Input: dimensioned drawing with shaded views. Units: mm. Origin: part minimum x, y, z. A direction names the side the tool comes from. Round coordinates to 2 decimals unless told otherwise and drop trailing zeros. Loops run counter-clockwise (first coordinate to the right, second up) from the corner with the lowest first, then second, coordinate; pieces in that order, holes last. Notation, with made-up numbers: M 43.5,-9 L 59.5,-9 A25 cw 59.5,6 Z; hole C 15,-35 d9. An arc over 180 degrees is marked long. Use one line per item in the form item = value. Start each with the question number.
Q1. Section query A-A, the plane x = 3.25. Output: boundary loops of the cut face in (y, z), and give its area (3 significant figures).
Q2. Section query C-C, the plane z = 1.85. Output: boundary loops of the cut face in (x, y).
Q3. First-contact query: P1, Ø0.7, axis at x = 3.5, z = 1, coming from the -Y side; P2, Ø0.7, axis at x = 3, z = 0.5, coming from the +Y side; P3, Ø1.5, axis at y = 3, z = 0.5, coming from the +X side; P4, Ø0.7, axis at y = 3.5, z = 1, coming from the -X side. Flat tips, straight axial feed; report the tip coordinate or a pass-through.
Q4. Section query D-D, the plane x = 5.75. Output: boundary loops of the cut face in (y, z), and give its area (3 significant figures).
Q5. Mould query, pull axis Y, two halves, no side actions, for the marked faces 6, 7, 8 and 9. Classes: pulls with the +Y half, pulls with the -Y half, needs draft (parallel to the pull), parting line crosses it, or undercut.
Q6. Access query for the marked faces 1, 2, 3, 4 and 5. Directions: +Z, -Z, +X, -X, +Y, -Y. A direction counts if a zero-diameter tool reaches every point of the face in a straight line with its end or side. Return the directions, or none.
Q7. Ray query, line 1 along Z through (x, y) = (2, 4.25); line 2 along Y through (x, z) = (3.75, 1.35); line 3 along X through (y, z) = (2.75, 1.5). Return the intervals inside material, ascending.
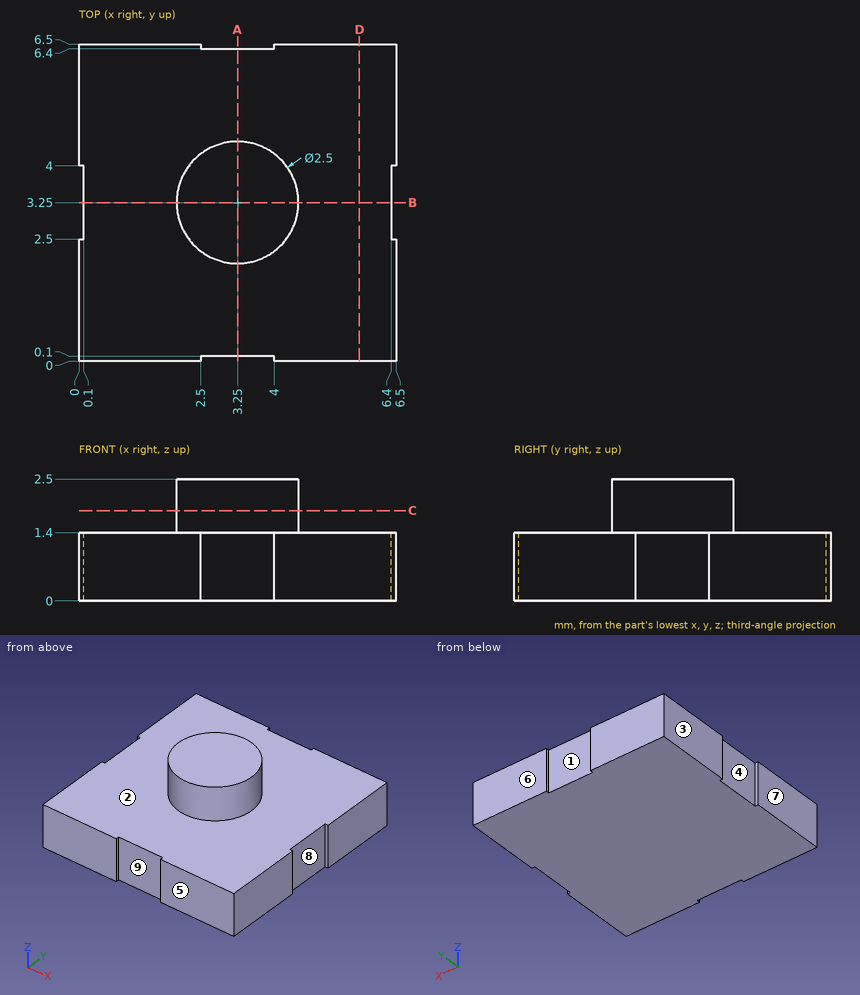
Results found:
q1.outline = M 0.1,0 L 6.4,0 L 6.4,1.4 L 4.5,1.4 L 4.5,2.5 L 2,2.5 L 2,1.4 L 0.1,1.4 Z
q1.area = 11.6 mm²
q2.outline = C 3.25,3.25 d2.5
q3.P1 = 0.1
q3.P2 = 6.4
q3.P3 = 6.5
q3.P4 = 0.1
q4.outline = M 0,0 L 6.5,0 L 6.5,1.4 L 0,1.4 Z
q4.area = 9.10 mm²
q5.face_6 = pulls with the +Y half
q5.face_7 = needs draft
q5.face_8 = undercut
q5.face_9 = pulls with the -Y half
q6.face_1 = +Z, -Z, +Y
q6.face_2 = +Z
q6.face_3 = +Z, -Z, -X, +Y, -Y
q6.face_4 = +Z, -Z, -X
q6.face_5 = +Z, -Z, +X, -X, -Y
q7.line_1 = 0 to 1.4
q7.line_2 = 0.1 to 6.4
q7.line_3 = 2.1 to 4.4
